from build123d import *

# Parameters (mm, degrees)
SKETCH_1_W          = 30
SKETCH_1_H          = 50
SKETCH_1_R          = 6.6
SKETCH_1_R_2        = 1.5
EXTRUDE_1_DEPTH     = 4
SKETCH_2_R          = 1.5
CUT_EXTRUDE_1_DEPTH = 59.446556785


with BuildPart() as part:
    # 草图1 → 凸台-拉伸1 (new body)
    with BuildSketch(Plane.XY):
        with Locations((15, 25)):
            Rectangle(SKETCH_1_W, SKETCH_1_H)
        with Locations((15, 27.5)):
            Circle(SKETCH_1_R, mode=Mode.SUBTRACT)
        with Locations((23.227241336, 32.25)):
            Circle(SKETCH_1_R_2, mode=Mode.SUBTRACT)
        with Locations((15, 18)):
            Circle(SKETCH_1_R_2, mode=Mode.SUBTRACT)
        with Locations((6.772758664, 32.25)):
            Circle(SKETCH_1_R_2, mode=Mode.SUBTRACT)
        with Locations((5, 47)):
            Circle(SKETCH_1_R_2, mode=Mode.SUBTRACT)
        with Locations((25, 47)):
            Circle(SKETCH_1_R_2, mode=Mode.SUBTRACT)
        with Locations((5, 3)):
            Circle(SKETCH_1_R_2, mode=Mode.SUBTRACT)
        with Locations((25, 3)):
            Circle(SKETCH_1_R_2, mode=Mode.SUBTRACT)
    extrude(amount=EXTRUDE_1_DEPTH)

    # 草图2 → 切除-拉伸1 (cut, through all)
    with BuildSketch(Plane.XY.offset(4)):
        with Locations((4, 42)):
            Circle(SKETCH_2_R)
        with Locations((26, 42)):
            Circle(SKETCH_2_R)
        with Locations((26, 8)):
            Circle(SKETCH_2_R)
        with Locations((4, 8)):
            Circle(SKETCH_2_R)
    extrude(amount=-CUT_EXTRUDE_1_DEPTH, mode=Mode.SUBTRACT)


solid = part.part
The listing builds one solid part. Answer for the finished solid, in the listing's coordinates (mm). Round coordinates to 2 decimals unless told otherwise and drop trailing zeros. Write each loop counter-clockwise with the first axis right and the second up, starting at its lowest first coordinate (ties: lowest second). Pieces come first, ordered by that corner, then holes. Notation, with made-up numbers: (19, -35) - (78, -35) arc R15 cw to (78, -21) - close; hole circle Ø3 at (-29, 9). An arc over 180 degrees is marked (long way). Use one line per item in the form item = value. Start each with the question number.
Item 1: Find the intervals of material crossed by line 1 (Y direction, x = 25, z = 1.55); line 2 (Y direction, x = 14.5, z = 2.1); line 3 (X direction, y = 22.5, z = 1.6), in increasing order. Write a range as [from, to].
Item 2: A cutting plane is placed at B-B (y = 3). Write down the section's boundary in (x, z).
Item 3: A cutting plane is placed at D-D (y = 18). Write down the section's boundary in (x, z).
Item 4: Determine the mould class of faces 1 (the cylindrical face through (7.465, 30.919, 1.972)), 2 (the flat face through (15, 20, 0)), 3 (the flat face through (15, 50, 2)) for opening direction Y: +Y half, -Y half, draft (parallel to the pull), parting line (faces both ways), or undercut.
Item 5: A cutting plane is placed at A-A (x = 15). Write down the section's boundary in (y, z).
Item 6: A cutting plane is placed at C-C (z = 3). Give the number of separate pieces and of enclosed holes in the cut face, plus the area to 3 significant figures.
Item 7: A flat-ended cylindrical pin translates along its axis: pin 1 Ø2.5 at (x, y) = (15, 18) entering from +Z. Find the tip coordinate at first contact, or state that the pin passes through.
The answers:
q1.line_1 = [0, 1.5], [4.5, 6.88], [9.12, 40.88], [43.12, 45.5], [48.5, 50]
q1.line_2 = [0, 16.59], [19.41, 20.92], [34.08, 50]
q1.line_3 = [0, 10.69], [19.31, 30]
q2.outline = (0, 0) - (3.5, 0) - (3.5, 4) - (0, 4) - close; (6.5, 0) - (23.5, 0) - (23.5, 4) - (6.5, 4) - close; (26.5, 0) - (30, 0) - (30, 4) - (26.5, 4) - close
q3.outline = (0, 0) - (13.5, 0) - (13.5, 4) - (0, 4) - close; (16.5, 0) - (30, 0) - (30, 4) - (16.5, 4) - close
q4.face_1 = undercut
q4.face_2 = draft
q4.face_3 = +Y half
q5.outline = (0, 0) - (16.5, 0) - (16.5, 4) - (0, 4) - close; (19.5, 0) - (20.9, 0) - (20.9, 4) - (19.5, 4) - close; (34.1, 0) - (50, 0) - (50, 4) - (34.1, 4) - close
q6.separate_pieces = 1
q6.enclosed_holes = 12
q6.area = 1,290 mm^2
q7.pin_1 = through
